Source: CAD feature listing. Evaluate the final solid. Frame: model axes, mm. A direction names the side the tool comes from. Round coordinates to 2 decimals unless told otherwise and drop trailing zeros. Loops run counter-clockwise (first coordinate to the right, second up) from the corner with the lowest first, then second, coordinate; pieces in that order, holes last. Notation, with made-up numbers: (-16.5, 54) -> (18.5, 54) arc R18 cw to (18.5, 61) -> close; hole circle Ø5 at (-32.5, 77). An arc over 180 degrees is marked (long way). Return JSON: item names as keys, results as strings. Group by question number.
```python
from build123d import *

# Parameters (mm, degrees)
SKETCH3_W               = 40
SKETCH3_H               = 30
BOSS_EXTRUDE1_DEPTH     = 2
SKETCH4_R               = 1.5
BOSS_EXTRUDE2_DEPTH     = 3
FILLET1_R               = 1
SKETCH8_W               = 20
SKETCH8_H               = 1
CUT_EXTRUDE2_DEPTH      = 2
FILLET3_R               = 1
SKETCH9_R               = 0.9
BOSS_EXTRUDE5_DEPTH     = 3
LPATTERN3_COUNT         = 2
LPATTERN3_PITCH         = 21
LPATTERN3_COUNT_DIR2    = 2
LPATTERN3_PITCH_DIR2    = 12.5
FILLET4_R               = 0.9
FILLET5_R               = 1
SKETCH11_R              = 1.05
CUT_EXTRUDE3_DEPTH      = 26.709920264
LPATTERN4_COUNT         = 2
LPATTERN4_PITCH         = 23
LPATTERN4_COUNT_DIR2    = 2
LPATTERN4_PITCH_DIR2    = 34
SKETCH12_W              = 40
SKETCH12_H              = 2.5
BOSS_EXTRUDE7_DEPTH     = 10
SKETCH13_R              = 2
CUT_EXTRUDE4_DEPTH      = 10
SKETCH14_W              = 2
SKETCH14_H              = 15
SKETCH14_W_2            = 10
SKETCH14_H_2            = 1.5
BOSS_EXTRUDE8_DEPTH     = 3.5
FILLET6_R               = 1
CUT_EXTRUDE5_DEPTH      = 44.874821937
CUT_EXTRUDE5_DEPTH_BACK = 44.874821937
SKETCH15_W              = 33.433671885
SKETCH15_H              = 17.879130682
SKETCH16_W              = 40
SKETCH16_H              = 15
BOSS_EXTRUDE9_DEPTH     = 2
FILLET8_R               = 1
FILLET9_R               = 1
FILLET10_R              = 0.25


with BuildPart() as part:
    # Sketch3 → Boss-Extrude1 (new body)
    with BuildSketch(Plane(origin=(0, 0, 0), x_dir=(1, 0, 0), z_dir=(0, 1, 0))):
        Rectangle(SKETCH3_W, SKETCH3_H)
    extrude(amount=BOSS_EXTRUDE1_DEPTH)

    # Sketch4 → Boss-Extrude2 (add)
    with BuildSketch(Plane(origin=(0, 2, 0), x_dir=(1, 0, 0), z_dir=(0, 1, 0))):
        with Locations(Location((-10.5, 9.25, 0), (0, 0, 270))):
            Circle(SKETCH4_R)
        with Locations(Location((10.5, 9.25, 0), (0, 0, 270))):
            Circle(SKETCH4_R)
        with Locations(Location((10.5, -3.25, 0), (0, 0, 270))):
            Circle(SKETCH4_R)
        with Locations(Location((-10.5, -3.25, 0), (0, 0, 270))):
            Circle(SKETCH4_R)
    extrude(amount=BOSS_EXTRUDE2_DEPTH)

    # Fillet1
    fillet1_edges = [part.edges().sort_by_distance(p)[0] for p in [
        (-20, 1, -15),
        (20, 1, -15),
    ]]
    fillet(fillet1_edges, radius=FILLET1_R)

    # Sketch8 → Cut-Extrude2 (cut)
    with BuildSketch(Plane(origin=(0, 2, 0), x_dir=(1, 0, 0), z_dir=(0, 1, 0))):
        with Locations((0, -14.5)):
            Rectangle(SKETCH8_W, SKETCH8_H)
    extrude(amount=-CUT_EXTRUDE2_DEPTH, mode=Mode.SUBTRACT)

    # Fillet3
    fillet3_edges = [part.edges().sort_by_distance(p)[0] for p in [
        (0, 0, 14),
        (0, 2, 14),
    ]]
    fillet(fillet3_edges, radius=FILLET3_R - 0.0001)  # a hair under: the kernel refuses the full size

    # Sketch9 → Boss-Extrude5 (add)
    with BuildSketch(Plane(origin=(0, 5, 0), x_dir=(1, 0, 0), z_dir=(0, 1, 0))):
        with Locations(Location((-10.5, 9.25, 0), (0, 0, 270))):
            Circle(SKETCH9_R)
    boss_extrude5 = extrude(amount=BOSS_EXTRUDE5_DEPTH)

    # LPattern3: Boss-Extrude5 2 × 2
    with Locations(*[(i * LPATTERN3_PITCH, 0, j * LPATTERN3_PITCH_DIR2) for i in range(LPATTERN3_COUNT) for j in range(LPATTERN3_COUNT_DIR2) if (i, j) != (0, 0)]):
        add(boss_extrude5)

    # Fillet4
    fillet4_edges = [part.edges().sort_by_distance(p)[0] for p in [
        (-10.5, 8, -10.15),
        (-10.5, 8, 2.35),
        (10.5, 8, -10.15),
        (10.5, 8, 2.35),
    ]]
    fillet(fillet4_edges, radius=FILLET4_R)

    # Fillet5
    fillet5_edges = [part.edges().sort_by_distance(p)[0] for p in [
        (20, 1, 15),
        (-20, 1, 15),
    ]]
    fillet(fillet5_edges, radius=FILLET5_R)

    # Sketch11 → Cut-Extrude3 (cut, through all)
    with BuildSketch(Plane(origin=(0, 2, 0), x_dir=(1, 0, 0), z_dir=(0, 1, 0))):
        with Locations(Location((-17, -11.5, 0), (0, 0, 270))):
            Circle(SKETCH11_R)
    cut_extrude3 = extrude(amount=-CUT_EXTRUDE3_DEPTH, mode=Mode.SUBTRACT)

    # LPattern4: Cut-Extrude3 2 × 2
    with Locations(*[(j * LPATTERN4_PITCH_DIR2, 0, -i * LPATTERN4_PITCH) for i in range(LPATTERN4_COUNT) for j in range(LPATTERN4_COUNT_DIR2) if (i, j) != (0, 0)]):
        add(cut_extrude3, mode=Mode.SUBTRACT)

    # Sketch12 → Boss-Extrude7 (add)
    with BuildSketch(Plane(origin=(0, 0, 0), x_dir=(-1, 0, 0), z_dir=(0, -1, 0))):
        with Locations((0, 2.25)):
            Rectangle(SKETCH12_W, SKETCH12_H)
    extrude(amount=BOSS_EXTRUDE7_DEPTH)

    # Sketch13 → Cut-Extrude4 (cut)
    with BuildSketch(Plane(origin=(0, 0, -3.5), x_dir=(-1, 0, 0), z_dir=(0, 0, -1))):
        with Locations((12, -5)):
            Circle(SKETCH13_R)
        with Locations((0, -5)):
            Circle(SKETCH13_R)
    extrude(amount=-CUT_EXTRUDE4_DEPTH, mode=Mode.SUBTRACT)

    # Sketch14 → Boss-Extrude8 (add)
    with BuildSketch(Plane(origin=(0, 2, 0), x_dir=(1, 0, 0), z_dir=(0, 1, 0))):
        with Locations((-17, 0)):
            Rectangle(SKETCH14_W, SKETCH14_H)
        with Locations((17, 0)):
            Rectangle(SKETCH14_W, SKETCH14_H)
        with Locations((0, 12.25)):
            Rectangle(SKETCH14_W_2, SKETCH14_H_2)
    extrude(amount=BOSS_EXTRUDE8_DEPTH)

    # Fillet6
    fillet6_edges = [part.edges().sort_by_distance(p)[0] for p in [
        (-16, 2, 0),
        (16, 2, 0),
        (0, 2, -11.5),
    ]]
    fillet(fillet6_edges, radius=FILLET6_R)

    # Sketch15 → Cut-Extrude5 (cut, two sides: drawn at the far end of the back side and taken through both)
    with BuildSketch(Plane.ZY.offset(20).offset(-CUT_EXTRUDE5_DEPTH_BACK)):
        with Locations((1.181680204, -8.939565341)):
            Rectangle(SKETCH15_W, SKETCH15_H)
    extrude(amount=CUT_EXTRUDE5_DEPTH + CUT_EXTRUDE5_DEPTH_BACK, mode=Mode.SUBTRACT)

    # Sketch16 → Boss-Extrude9 (add)
    with BuildSketch(Plane.XZ):
        Rectangle(SKETCH16_W, SKETCH16_H)
    extrude(amount=BOSS_EXTRUDE9_DEPTH)

    # Fillet8
    fillet8_edges = [part.edges().sort_by_distance(p)[0] for p in [
        (0, 0, -7.5),
    ]]
    fillet(fillet8_edges, radius=FILLET8_R)

    # Fillet9
    fillet9_edges = [part.edges().sort_by_distance(p)[0] for p in [
        (0, 0, 7.5),
    ]]
    fillet(fillet9_edges, radius=FILLET9_R)

    # Fillet10
    fillet10_edges = [part.edges().sort_by_distance(p)[0] for p in [
        (0, -2, 7.5),
        (0, -2, -7.5),
    ]]
    fillet(fillet10_edges, radius=FILLET10_R)


solid = part.part
```
(1) Set-up query: faces 5 (the face through (-16, 4, 0)), 6 (the face through (0, 2, 0)), 7 (the face through (0.14, 0.285, 13.699)), 8 (the face through (17, 4, 7.5)), 9 (the face through (0, 0, -12)). Return all of +Z, -Z, +X, -X, +Y, -Y with unobstructed straight access to the full face (end or side cutting, diameter ignored); none if empty.
(2) Mould query, pull axis Z, two halves, no side actions, for faces 1 (the face through (11.39, 6.04, -9.37)), 2 (the face through (-18, 4, 0)), 3 (the face through (0.14, 1.715, 13.699)), 4 (the face through (-9.61, 6.04, 3.13)). Classes: released by +Z, released by -Z, zero draft, split by the parting line, or undercut.
(3) Cut plane A-A (x = 17). Return loops of the section in (y, z).
(4) Cut plane C-C (y = 4). Return loops of the section in (x, z).
(5) Ray query, line 1 (X direction, y = 1.2, z = 11.5); line 2 (Y direction, x = -5, z = 7); line 3 (Y direction, x = -2.5, z = -9.5). Return the intervals inside material, ascending.
(6) Pin query (flat end, axial travel): pin 1 (1.6 mm diameter, centred on y = 1.5, z = 14.5, fed in from +X); pin 2 (1.8 mm diameter, centred on x = 0.5, y = 3, fed in from -Z); pin 3 (1 mm diameter, centred on x = -13, z = -0.5, fed in from +Y); pin 4 (2.5 mm diameter, centred on x = 17, z = 11.5, fed in from -Y). Return the tip coordinate at first contact, or that it passes through.
(7) Cut plane B-B (z = 11.5). Return loops of the section in (x, y).
Answers follow:
{
 "1": {"face 5": "+Z, -Z, +Y", "face 6": "+Y", "face 7": "+Z, -Y", "face 8": "+Z, +X, -X, +Y", "face 9": "-Z, +X, -X, -Y"},
 "2": {"face 1": "undercut", "face 2": "zero draft", "face 3": "released by +Z", "face 4": "undercut"},
 "3": {"outline": "(-2, -7.25) arc R0.25 ccw to (-1.75, -7.5) -> (-1, -7.5) arc R1 cw to (0, -8.5) -> (0, -10.45) -> (2, -10.45) -> (2, -7.5) -> (5.5, -7.5) -> (5.5, 7.5) -> (2, 7.5) -> (2, 10.45) -> (0, 10.45) -> (0, 8.5) arc R1 cw to (-1, 7.5) -> (-1.75, 7.5) arc R0.25 ccw to (-2, 7.25) -> close; (0, -15) -> (2, -15) -> (2, -12.55) -> (0, -12.55) -> close; (0, 12.55) -> (2, 12.55) -> (2, 15) -> (0, 15) -> close"},
 "4": {"outline": "(-18, -7.5) -> (-16, -7.5) -> (-16, 7.5) -> (-18, 7.5) -> close; circle Ø3 at (-10.5, -9.25); circle Ø3 at (-10.5, 3.25); (-5, -13) -> (5, -13) -> (5, -11.5) -> (-5, -11.5) -> close; circle Ø3 at (10.5, -9.25); circle Ø3 at (10.5, 3.25); (16, -7.5) -> (18, -7.5) -> (18, 7.5) -> (16, 7.5) -> close"},
 "5": {"line 1": "-20 to -18.05, -15.95 to 15.95, 18.05 to 20", "line 2": "-2 to 2", "line 3": "0 to 2"},
 "6": {"pin 1": "x = 20", "pin 2": "z = -13", "pin 3": "y = 2", "pin 4": "y = 0"},
 "7": {"outline": "(-20, 0) -> (-18.05, 0) -> (-18.05, 2) -> (-20, 2) -> close; (-15.95, 0) -> (15.95, 0) -> (15.95, 2) -> (-15.95, 2) -> close; (18.05, 0) -> (20, 0) -> (20, 2) -> (18.05, 2) -> close"}
}
